Input: part model. Units: mm. Frame: model coordinates. Coordinates: 2 decimals unless noted, no trailing zeros. Use one line per item in the form item = value. Start each with the question number.
1) Draft query along Z for faces 1 (the flat face through (-1, 1.588, -11)), 2 (the cylindrical face through (-24.567, 0.022, 7.464)), 3 (the flat face through (-57.91, 0.02, 37.72)), 4 (the cylindrical face through (-30.2, 0, 48.9)). Return one class per face: pulls with the +Z half, pulls with the -Z half, needs draft (parallel to the pull), parting line crosses it, or undercut.
2) Section query A-A on y = -0.8. Count the separate pieces of the cut face and the enclosed holes in it, then the cut area to 3 significant figures.
3) Pin query (flat end, axial travel): pin 1 (3 mm diameter, centred on x = 26, z = 6.55, fed in from -Y); pin 2 (1.6 mm diameter, centred on y = 0.5, z = 63, fed in from -X); pin 3 (1.6 mm diameter, centred on y = -1, z = 62.5, fed in from +X); pin 4 (1.6 mm diameter, centred on y = 1, z = 29.5, fed in from -X). Return the tip coordinate at first contact, or that it passes through.
4) Ray query, line 1 along Z through (x, y) = (-36.5, 0.4); line 2 along X through (y, z) = (-0.15, -19.8); line 3 along X through (y, z) = (-0.25, 5). Return the intervals inside material, ascending.
from build123d import *

# Parameters (mm, degrees)
BOSS_EXTRUDE4_DEPTH  = 1.5875
M3_CLEARANCE_HOLE3_D = 3
M3_CLEARANCE_HOLE1_D = 3.1
M3_CLEARANCE_HOLE4_D = 2.95
M3_CLEARANCE_HOLE2_D = 3.1
BOSS_EXTRUDE6_DEPTH  = 3.175
FILLET1_R            = 2
FILLET3_R            = 1
FILLET6_R            = 0.5
CUT_EXTRUDE4_DEPTH   = 10
SKETCH29_R           = 1.75
CUT_EXTRUDE5_DEPTH   = 10
SKETCH31_R           = 1.7
CUT_EXTRUDE7_DEPTH   = 10


with BuildPart() as part:
    # Sketch1 → Boss-Extrude4 (new, symmetric)
    with BuildSketch(Plane(origin=(0, 0, 0), x_dir=(1, 0, 0), z_dir=(0, 1, 0))):
        with BuildLine():
            Line((-62.799553621, 32.496136604), (-73.969425011, 32.691107434))
            Line((-73.969425011, 32.691107434), (-77.053684287, 35.88495141))
            ThreePointArc((-77.053684287, 35.88495141), (-84.36642289, 10.358894189), (-83.446216027, -16.178041625))
            Line((-83.446216027, -16.178041625), (-79.680911643, -13.825218315))
            Line((-79.680911643, -13.825218315), (-69.484649137, -16.179210996))
            Line((-69.484649137, -16.179210996), (-43.894490772, -57.132025032))
            Line((-43.894490772, -57.132025032), (-43.894490772, -64.826600275))
            Line((-43.894490772, -64.826600275), (-43.094490772, -64.826600275))
            Line((-43.094490772, -64.826600275), (-34, -64.826600275))
            Line((-34, -64.826600275), (-34, -59.55))
            Line((-34, -59.55), (-34, -58.55))
            Line((-34, -58.55), (-20, -58.55))
            Line((-20, -58.55), (-19.859459165, -59.55))
            Line((-19.859459165, -59.55), (19.859459165, -59.55))
            Line((19.859459165, -59.55), (20, -58.55))
            Line((20, -58.55), (34, -58.55))
            Line((34, -58.55), (34, -59.55))
            Line((34, -59.55), (34, -64.826600275))
            Line((34, -64.826600275), (43.094490772, -64.826600275))
            Line((43.094490772, -64.826600275), (43.894490772, -64.826600275))
            Line((43.894490772, -64.826600275), (43.894490772, -57.132025032))
            Line((43.894490772, -57.132025032), (69.484649137, -16.179210996))
            Line((69.484649137, -16.179210996), (79.680911643, -13.825218315))
            Line((79.680911643, -13.825218315), (83.446216027, -16.178041625))
            ThreePointArc((83.446216027, -16.178041625), (84.610662337, -8.126242604), (85, 0))
            ThreePointArc((85, 0), (82.98964744, 18.377116688), (77.053684287, 35.88495141))
            Line((77.053684287, 35.88495141), (73.969425011, 32.691107434))
            Line((73.969425011, 32.691107434), (62.799553621, 32.496136604))
            Line((62.799553621, 32.496136604), (30.284668021, 63.895396642))
            Line((30.284668021, 63.895396642), (30.089697191, 75.065268032))
            Line((30.089697191, 75.065268032), (33.173956467, 78.259112008))
            ThreePointArc((33.173956467, 78.259112008), (0, 85), (-33.173956467, 78.259112008))
            Line((-33.173956467, 78.259112008), (-30.089697191, 75.065268032))
            Line((-30.089697191, 75.065268032), (-30.284668021, 63.895396642))
            Line((-30.284668021, 63.895396642), (-62.799553621, 32.496136604))
        make_face()
    extrude(amount=BOSS_EXTRUDE4_DEPTH, both=True)

    # M3 Clearance Hole3 (through all)
    with Locations(Plane(origin=(0, -1.5875, 0), x_dir=(-1, 0, 0), z_dir=(0, -1, 0))):
        with Locations((36.5, -50), (36.5, -38), (-36.5, -50), (-36.5, -38)):
            Hole(M3_CLEARANCE_HOLE3_D / 2)

    # M3 Clearance Hole1 (through all)
    with Locations(Plane(origin=(0, 1.5875, 0), x_dir=(1, 0, 0), z_dir=(0, 1, 0))):
        with Locations((-78.542321426, -8.49139241), (78.542321426, -8.49139241), (74.155025063, 27.240269049), (-74.155025063, 27.240269049)):
            Hole(M3_CLEARANCE_HOLE1_D / 2)

    # M3 Clearance Hole4 (through all)
    with Locations(Plane(origin=(0, -1.5875, 0), x_dir=(-1, 0, 0), z_dir=(0, -1, 0))):
        with Locations((-67.099301622, -15.278865202), (-50.141885166, -42.416404279), (-61.062544382, 30.698137949), (-38.043670771, 52.927205804), (50.141885166, -42.416404279), (67.099301622, -15.278865202), (38.043670771, 52.927205804), (61.062544382, 30.698137949)):
            Hole(M3_CLEARANCE_HOLE4_D / 2)

    # M3 Clearance Hole2 (through all)
    with Locations(Plane(origin=(0, 1.5875, 0), x_dir=(1, 0, 0), z_dir=(0, 1, 0))):
        with Locations((27, 76.497766718), (-27, 76.497766718)):
            Hole(M3_CLEARANCE_HOLE2_D / 2)

    # Sketch22 → Boss-Extrude6 (add)
    with BuildSketch(Plane(origin=(0, 1.5875, 0), x_dir=(1, 0, 0), z_dir=(0, 1, 0))):
        Polygon((65.061950694, 32.535626892), (30.245177733, 66.157793715), (30.284668021, 63.895396642), (62.799553621, 32.496136604), align=None)
        Polygon((-30.284668021, 63.895396642), (-30.245177733, 66.157793715), (-65.061950694, 32.535626892), (-62.799553621, 32.496136604), align=None)
        Polygon((43.894490772, -60.151352895), (71.689396914, -15.670204865), (69.484649137, -16.179210996), (43.894490772, -57.132025032), align=None)
        Polygon((-69.484649137, -16.179210996), (-71.689396914, -15.670204865), (-43.894490772, -60.151352895), (-43.894490772, -57.132025032), align=None)
    extrude(amount=-BOSS_EXTRUDE6_DEPTH)

    # Fillet1
    fillet1_edges = [part.edges().sort_by_distance(p)[0] for p in [
        (-30.245177733, 0.79375, -66.157793715),
        (-65.061950694, 0.79375, -32.535626892),
        (-71.689396914, 0.79375, 15.670204865),
        (-43.894490772, 0.79375, 60.151352895),
        (43.894490772, -0.79375, 60.151352895),
        (71.689396914, -0.79375, 15.670204865),
        (65.061950694, 0.79375, -32.535626892),
        (30.245177733, -0.79375, -66.157793715),
        (30.089697191, -0.79375, -75.065268032),
        (73.969425011, -0.79375, -32.691107434),
        (79.680911643, -0.79375, 13.825218315),
        (-79.680911643, -0.79375, 13.825218315),
        (-73.969425011, -0.79375, -32.691107434),
        (-30.089697191, -0.79375, -75.065268032),
    ]]
    fillet(fillet1_edges, radius=FILLET1_R)

    # Fillet3
    fillet3_edges = [part.edges().sort_by_distance(p)[0] for p in [
        (33.173956467, -0.79375, -78.259112008),
        (77.053684287, 0.79375, -35.88495141),
        (83.446216027, -0.79375, 16.178041625),
        (43.894490772, -0.79375, 64.826600275),
        (34, 0.79375, 64.826600275),
        (34, -0.79375, 58.55),
        (-34, -0.79375, 58.55),
        (-34, 0.79375, 64.826600275),
        (-43.894490772, -0.79375, 64.826600275),
        (-83.446216027, -0.79375, 16.178041625),
        (-77.053684287, -0.79375, -35.88495141),
        (-33.173956467, -0.79375, -78.259112008),
    ]]
    fillet(fillet3_edges, radius=FILLET3_R - 0.0001)  # a hair under: the kernel refuses the full size

    # Fillet6
    fillet6_edges = [part.edges().sort_by_distance(p)[0] for p in [
        (20, -0.79375, 58.55),
        (19.859459165, -0.79375, 59.55),
        (-19.859459165, 0.79375, 59.55),
        (-20, 0.79375, 58.55),
    ]]
    fillet(fillet6_edges, radius=FILLET6_R)

    # Sketch28 → Cut-Extrude4 (cut)
    with BuildSketch(Plane(origin=(0, 1.5875, 0), x_dir=(1, 0, 0), z_dir=(0, 1, 0))):
        with BuildLine():
            Line((-26.25, -9.55), (-26.25, -59.55))
            Line((-26.25, -59.55), (26.25, -59.55))
            Line((26.25, -59.55), (26.25, -9.55))
            Line((26.25, -9.55), (21.2, -9.55))
            Line((21.2, -9.55), (21.2, -1.5))
            Line((21.2, -1.5), (4.195235393, -1.5))
            ThreePointArc((4.195235393, -1.5), (0, 2.5), (-4.195235393, -1.5))
            Line((-4.195235393, -1.5), (-21.2, -1.5))
            Line((-21.2, -1.5), (-21.2, -9.55))
            Line((-21.2, -9.55), (-26.25, -9.55))
        make_face()
    extrude(amount=-CUT_EXTRUDE4_DEPTH, mode=Mode.SUBTRACT)

    # Sketch29 → Cut-Extrude5 (cut)
    with BuildSketch(Plane(origin=(0, 1.5875, 0), x_dir=(1, 0, 0), z_dir=(0, 1, 0))):
        with Locations(Location((30.25, -50.65, 0), (0, 0, 270))):
            Circle(SKETCH29_R)
        with Locations(Location((-30.25, -50.65, 0), (0, 0, 270))):
            Circle(SKETCH29_R)
    extrude(amount=-CUT_EXTRUDE5_DEPTH, mode=Mode.SUBTRACT)

    # Sketch31 → Cut-Extrude7 (cut)
    with BuildSketch(Plane(origin=(0, 1.5875, 0), x_dir=(1, 0, 0), z_dir=(0, 1, 0))):
        with Locations(Location((-26, -6.55, 0), (0, 0, 270))):
            Circle(SKETCH31_R)
        with Locations(Location((26, -6.55, 0), (0, 0, 270))):
            Circle(SKETCH31_R)
        with Locations(Location((-26, 19.8, 0), (0, 0, 270))):
            Circle(SKETCH31_R)
        with Locations(Location((26, 19.8, 0), (0, 0, 270))):
            Circle(SKETCH31_R)
    extrude(amount=-CUT_EXTRUDE7_DEPTH, mode=Mode.SUBTRACT)


solid = part.part
Answers below:
q1.face_1 = needs draft
q1.face_2 = undercut
q1.face_3 = pulls with the +Z half
q1.face_4 = undercut
q2.separate_pieces = 1
q2.enclosed_holes = 24
q2.area = 14,300 mm^2
q3.pin_1 = through
q3.pin_2 = -43.89
q3.pin_3 = 43.89
q3.pin_4 = -63.55
q4.line_1 = -60.12 to 36.5, 39.5 to 48.5, 51.5 to 64.83
q4.line_2 = -82.66 to -27.7, -24.3 to 24.3, 27.7 to 82.66
q4.line_3 = -84.85 to -26.7, -25.3 to -21.2, 21.2 to 25.3, 26.7 to 84.85
